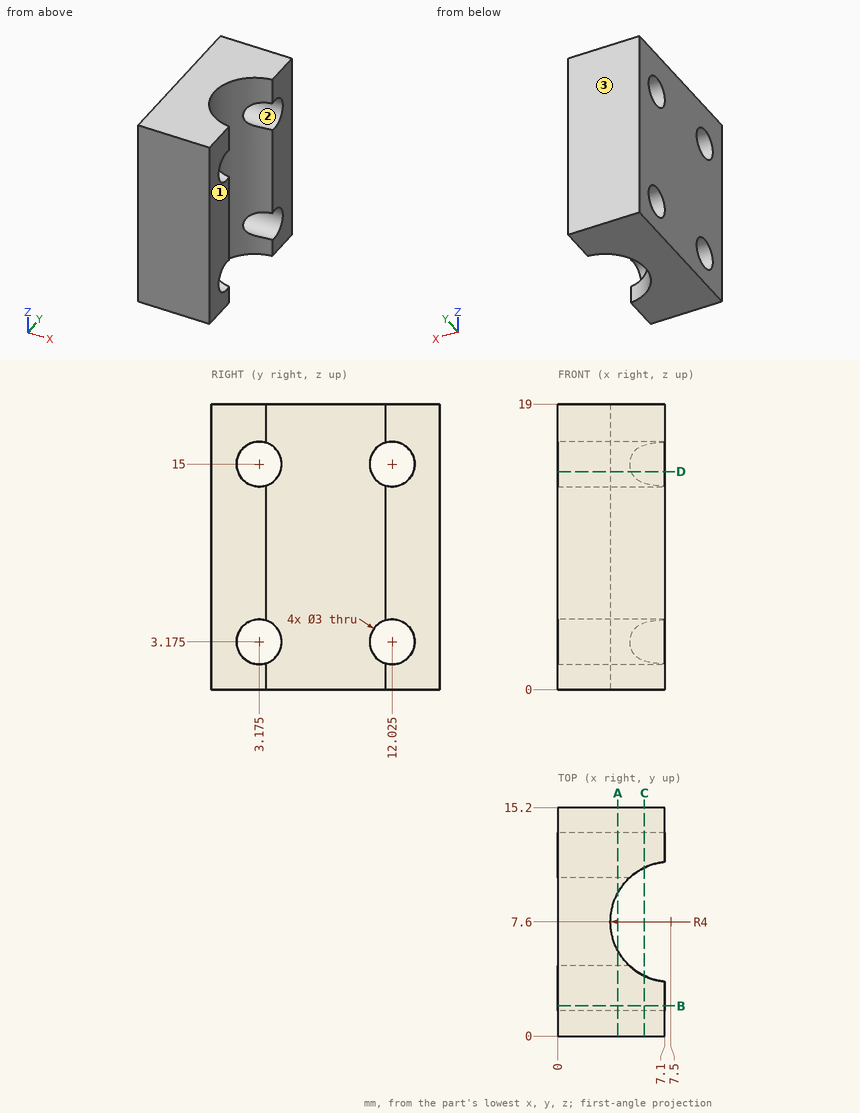
Study the drawing (mm; zero at the part's minimum x, y, z) and answer. Give positions to 0.01 mm unless a question says otherwise; leave off trailing zeros. Loops run counter-clockwise (first coordinate to the right, second up) from the corner with the lowest first, then second, coordinate; pieces in that order, holes last. Notation, with made-up numbers: (-39, 88) - (14, 88) arc R27 cw to (14, 119) - close; hole circle Ø11 at (78.5, 88.25). An arc over 180 degrees is marked (long way). Answer as CSV lines item,"result". Start each with the question number.
1) Find section D-D (z = 14.5). Write down the section's boundary in (x, y).
2) Find section B-B (y = 2). Write down the section's boundary in (x, z).
3) Find section A-A (x = 4). Write down the section's boundary in (y, z) (1 decimal), then the cut area to 3 significant figures.
4) Straight lines are drawn through the part: L1, parallel to Y at x = 2.25, z = 15 (3 decimals); L2, parallel to Z at x = 2.5, y = 12; L3, parallel to Y at x = 3.25, z = 16. For each, find the intervals that lie inside material, in ascending order. Write a range as from..to.
5) This flat-tipped pin is pushed along its axis until it touches: pin 1 Ø2.5 at (y, z) = (3.175, 15) entering from +X. Where does it stop, or does it pass through?
6) Find section C-C (x = 5.75). Write down the section's boundary in (y, z) (3 decimals), then the cut area to 3 significant figures.
7) Determine the mould class of the marked faces 1, 2 and 3 for opening direction Y: released by +Y, released by -Y, zero draft, split by the parting line, or undercut.
Findings below:
1,outline,"(0, 0) - (7.1, 0) - (7.1, 1.76) - (0, 1.76) - close; (0, 4.59) - (4.87, 4.59) arc R4 cw to (4.87, 10.61) - (0, 10.61) - close; (0, 13.44) - (7.1, 13.44) - (7.1, 15.2) - (0, 15.2) - close"
2,outline,"(0, 0) - (7.1, 0) - (7.1, 2.24) - (0, 2.24) - close; (0, 4.11) - (7.1, 4.11) - (7.1, 14.07) - (0, 14.07) - close; (0, 15.93) - (7.1, 15.93) - (7.1, 19) - (0, 19) - close"
3,outline,"(0, 0) - (5.7, 0) - (5.7, 19) - (0, 19) - close; (9.5, 0) - (15.2, 0) - (15.2, 19) - (9.5, 19) - close; hole circle Ø3 at (3.2, 3.2); hole circle Ø3 at (3.2, 15); hole circle Ø3 at (12, 3.2); hole circle Ø3 at (12, 15)"
3,area,"187 mm^2"
4,L1,"0..1.675, 4.675..10.525, 13.525..15.2"
4,L2,"0..1.68, 4.67..13.5, 16.5..19"
4,L3,"0..2.06, 4.29..10.91, 13.14..15.2"
5,pin 1,"through"
6,outline,"(0, 0) - (4.003, 0) - (4.003, 1.924) arc R1.5 cw (long way) to (4.003, 4.426) - (4.003, 13.749) arc R1.5 cw (long way) to (4.003, 16.251) - (4.003, 19) - (0, 19) - close; (11.197, 0) - (15.2, 0) - (15.2, 19) - (11.197, 19) - (11.197, 16.251) arc R1.5 cw (long way) to (11.197, 13.749) - (11.197, 4.426) arc R1.5 cw (long way) to (11.197, 1.924) - close"
6,area,"129 mm^2"
7,face 1,"zero draft"
7,face 2,"undercut"
7,face 3,"released by +Y"
